For this review, take the finished solid that the model builds, in its own axes (mm). Face numbers are marked on the shaded views. A direction names the side the tool comes from. Give positions to 0.01 mm unless a question says otherwise; leave off trailing zeros. Order: outer loops, then holes, each group sorted by start corner. A loop starts at its lowest first (then second) coordinate and runs counter-clockwise, first axis right, second up. Notation, with made-up numbers: M 81.5,22.5 L 121.5,22.5 A22 ccw 121.5,41.5 Z; hole C 36.5,47.25 d4. An arc over 180 degrees is marked long. Use CSV: the item, a comma, the result in double quotes. Start each with the question number.
(1) Clearance check with flat-ended pins moving along their axes: P1, Ø2, axis at y = 277, z = 12.5, coming from the +X side; P2, Ø3, axis at y = 274.5, z = 13, coming from the -X side; P3, Ø1.5, axis at y = 277.5, z = 18, coming from the +X side. State where each tip first meets the part, or that it passes through.
(2) Consider section B-B (x = 268). Write out the cut boundary in (y, z).
(3) Consider section A-A (y = 272). Write out the cut boundary in (x, z), and give its area (3 significant figures).
(4) Tool access review of the marked faces 1, 2, 3, 4 and 5: name each direction out of +Z, -Z, +X, -X, +Y, -Y from which nothing blocks a thin tool from reaching the whole face with its end or side.
(5) Consider section C-C (y = 277.5). Write out the cut boundary in (x, z).
(6) Wall thickness on L1, parallel to Y at x = 289.5, z = 19.75; L2, parallel to X at y = 263.5, z = 20.75; L3, parallel to Y at x = 286, z = 21: over which ranges is each line inside the solid? List them lowest first. Write a range as from..to.
(7) Consider section D-D (x = 261.5). Write out the cut boundary in (y, z).
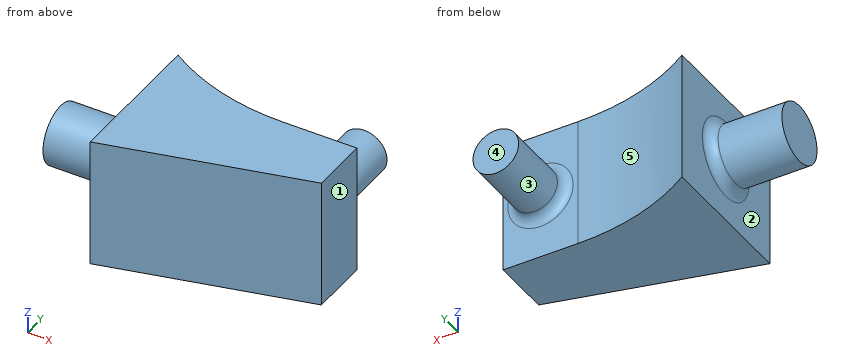
```python
from build123d import *

# Parameters (mm, degrees)
BOSS_EXTRUDE1_DEPTH = 26.416
SKETCH5_R           = 4.656567863
BOSS_EXTRUDE2_DEPTH = 15.24
SKETCH6_R           = 6
BOSS_EXTRUDE3_DEPTH = 15
FILLET1_R           = 2
FILLET2_R           = 2


with BuildPart() as part:
    # Sketch4 → Boss-Extrude1 (new body)
    with BuildSketch(Plane.XY):
        with BuildLine():
            Line((253.405334172, 274.985392586), (253.405334172, 244.985392586))
            Line((253.405334172, 244.985392586), (294.436722218, 255.22168408))
            Line((294.436722218, 255.22168408), (294.436722218, 267.343480441))
            Line((294.436722218, 267.343480441), (279.196722218, 267.343480441))
            ThreePointArc((279.196722218, 267.343480441), (265.746866098, 269.294144182), (253.405334172, 274.985392586))
        make_face()
    extrude(amount=BOSS_EXTRUDE1_DEPTH)

    # Sketch5 → Boss-Extrude2 (add)
    with BuildSketch(Plane(origin=(0, 267.343480441, 0), x_dir=(1, 0, 0), z_dir=(0, 1, 0))):
        with Locations(Location((286.816722218, -13.208, 0), (0, 0, 90))):
            Circle(SKETCH5_R)
    extrude(amount=BOSS_EXTRUDE2_DEPTH)

    # Sketch6 → Boss-Extrude3 (add)
    with BuildSketch(Plane.ZY.offset(-253.405334172)):
        with Locations((13.208, 259.985392586)):
            Circle(SKETCH6_R)
    extrude(amount=BOSS_EXTRUDE3_DEPTH)

    # Fillet1
    fillet1_edges = [part.edges().sort_by_distance(p)[0] for p in [
        (253.405334172, 259.985392586, 7.208),
    ]]
    fillet(fillet1_edges, radius=FILLET1_R)

    # Fillet2
    fillet2_edges = [part.edges().sort_by_distance(p)[0] for p in [
        (286.816722218, 267.343480441, 17.864567863),
    ]]
    fillet(fillet2_edges, radius=FILLET2_R)


solid = part.part
```
Check result:
1,P1,"stops at x = 291.47"
1,P2,"stops at x = 253.41"
1,P3,"stops at x = 289.13"
2,outline,"M 248.63,0 L 268.69,0 L 268.69,26.42 L 248.63,26.42 Z"
3,outline,"M 253.41,0 L 258.72,0 L 258.72,26.42 L 253.41,26.42 Z; C 286.82,13.21 d9.31"
3,area,"209 mm^2"
4,face 1,"+Z, -Z, +X, +Y, -Y"
4,face 2,"-X"
4,face 3,"+Y"
4,face 4,"+Z, -Z, +X, -X, +Y"
4,face 5,"+Z, -Z, +Y"
5,outline,"C 286.82,13.21 d9.31"
6,L1,"y = 253.99..267.34"
6,L2,"x = 253.41..294.44"
6,L3,"y = 253.12..267.34"
7,outline,"M 247,0 L 270.78,0 L 270.78,26.42 L 247,26.42 Z"
